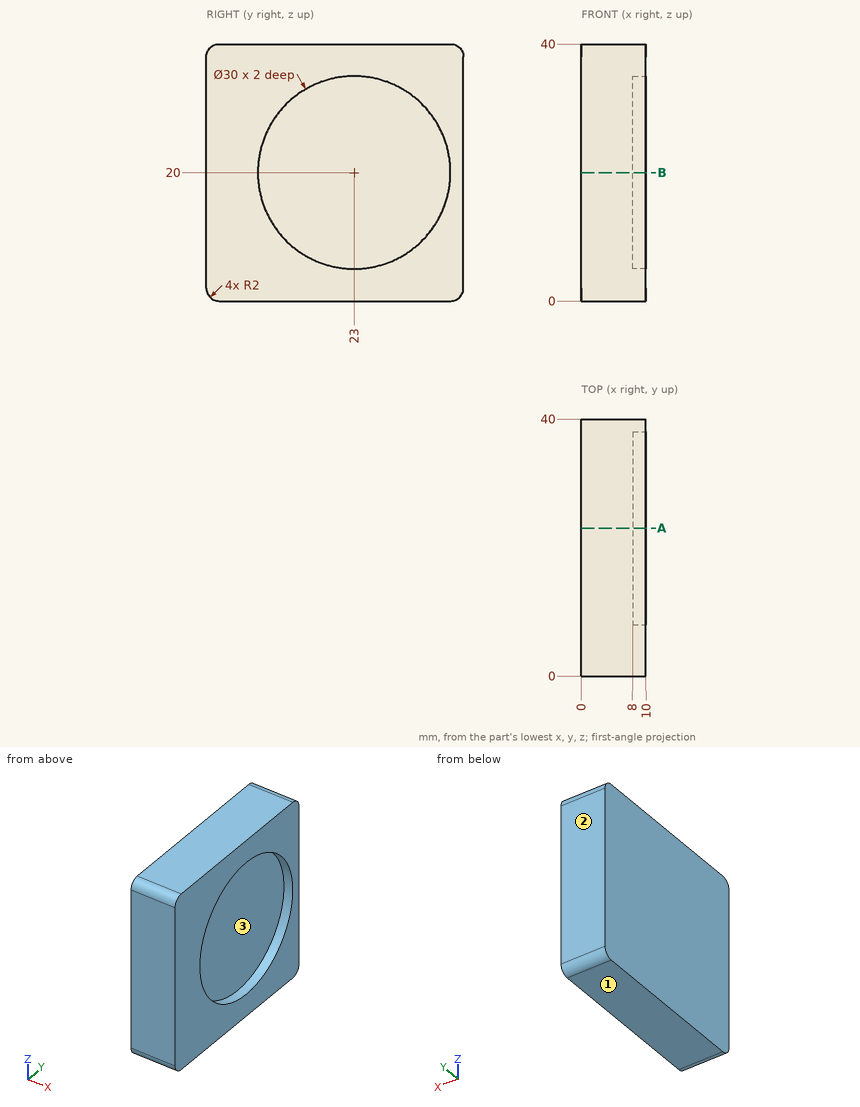
Print and shaded views of the part. All mm, measured from the part's lowest x, y and z. Give positions to 0.01 mm unless a question says otherwise; leave off trailing zeros. Order: outer loops, then holes, each group sorted by start corner. A loop starts at its lowest first (then second) coordinate and runs counter-clockwise, first axis right, second up. Notation, with made-up numbers: (-23.75, -28) - (18.25, -28) arc R15 ccw to (18.25, -11) - close; hole circle Ø6 at (12, -11.5). An arc over 180 degrees is marked (long way). One line per item, written item: value.
Item 1: Wall check: line 1 (Y direction, x = 8.95, z = 20); line 2 (X direction, y = 21, z = 21); line 3 (Y direction, x = 8.5, z = 23). Give the ranges that are in metal, low to high.
Response values:
line 1: 0 to 8, 38 to 40
line 2: 0 to 8
line 3: 0 to 8.3, 37.7 to 40
Item 2: Pin check, flat tip, straight feed: pin 1 Ø2 at (y, z) = (22, 33) entering from +X. Stop position of the tip, or through.
Response values:
pin 1: x = 8
Item 3: Two-plate mould, pull along Z, no slides. Class the marked faces 1, 2 and 3: released by +Z, released by -Z, zero draft, split by the parting line, or undercut.
Response values:
face 1: released by -Z
face 2: zero draft
face 3: undercut
Item 4: Slice it at B-B (z = 20). List the corners of the cut face in (x, y), then the cut area to 3 significant figures.
Response values:
outline: (0, 0) - (10, 0) - (10, 8) - (8, 8) - (8, 38) - (10, 38) - (10, 40) - (0, 40) - close
area: 340 mm2
Item 5: Slice it at A-A (y = 23). List the corners of the cut face in (x, z).
Response values:
outline: (0, 0) - (10, 0) - (10, 5) - (8, 5) - (8, 35) - (10, 35) - (10, 40) - (0, 40) - close
